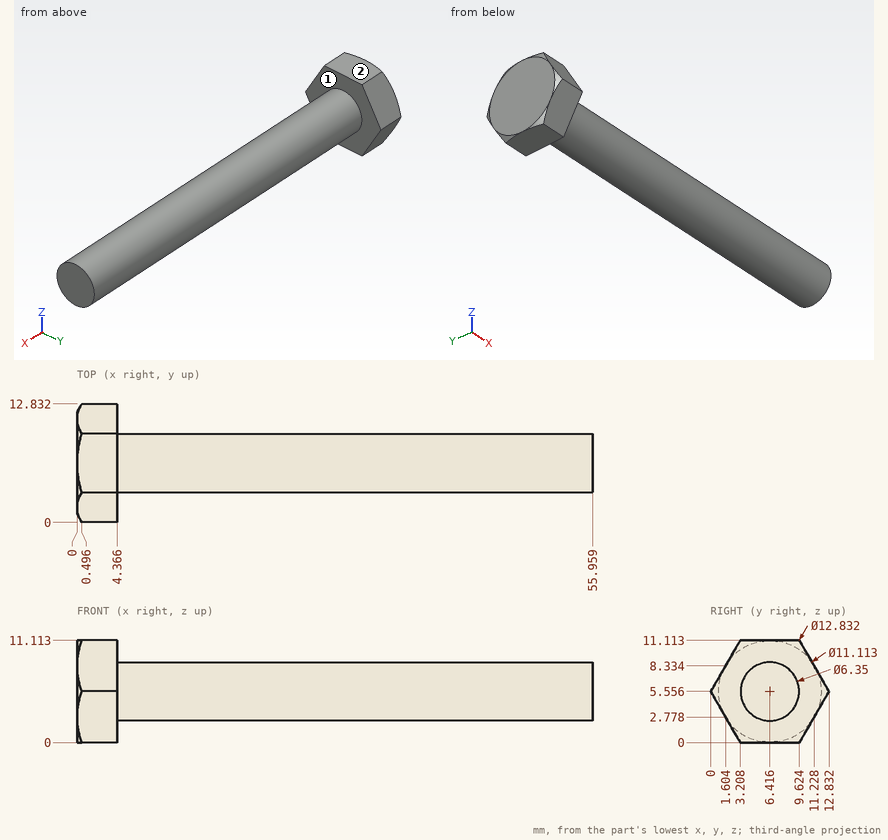
Can you work these out from the drawing? Everything is in mm from the part's minimum corner. A direction names the side the tool comes from. Round coordinates to 2 decimals unless told otherwise and drop trailing zeros. Answer in a Markdown table with one row per item.
Item 1: Will these pins go through, and if not, where does the flat tip stop? P1, Ø2, axis at x = 12.5, z = 9, coming from the -Y side; P2, Ø1, axis at x = 49, y = 2, coming from the +Z side; P3, Ø4, axis at x = 20.5, z = 2, coming from the -Y side; P4, Ø2, axis at x = 45, y = 9.5, coming from the -Z side.
Answer block:
| item | result |
|---|---|
| P1 | y = 4.39 |
| P2 | through |
| P3 | y = 3.65 |
| P4 | z = 3.16 |
Item 2: If I drill on probe 1 along X at (y, z) = (8, 1.25) (1 decimal); probe 2 along Y at (x, z) = (27, 5.5); probe 3 along Y at (x, z) = (23, 7.25), over which ranges is the centre line in solid material (lowest first)?
Answer block:
| item | result |
|---|---|
| probe 1 | 0 to 4.4 |
| probe 2 | 3.24 to 9.59 |
| probe 3 | 3.73 to 9.1 |
Item 3: On a 3-axis mill with a long thin cutter (end or side, diameter ignored), from which of +Z, -Z, +X, -X, +Y, -Y can I reach the whole of each face in a straight line? I mean the marked faces 1 and 2. Say none if no direction works.
Answer block:
| item | result |
|---|---|
| face 1 | +X |
| face 2 | +Z, +X, -X, +Y, -Y |
